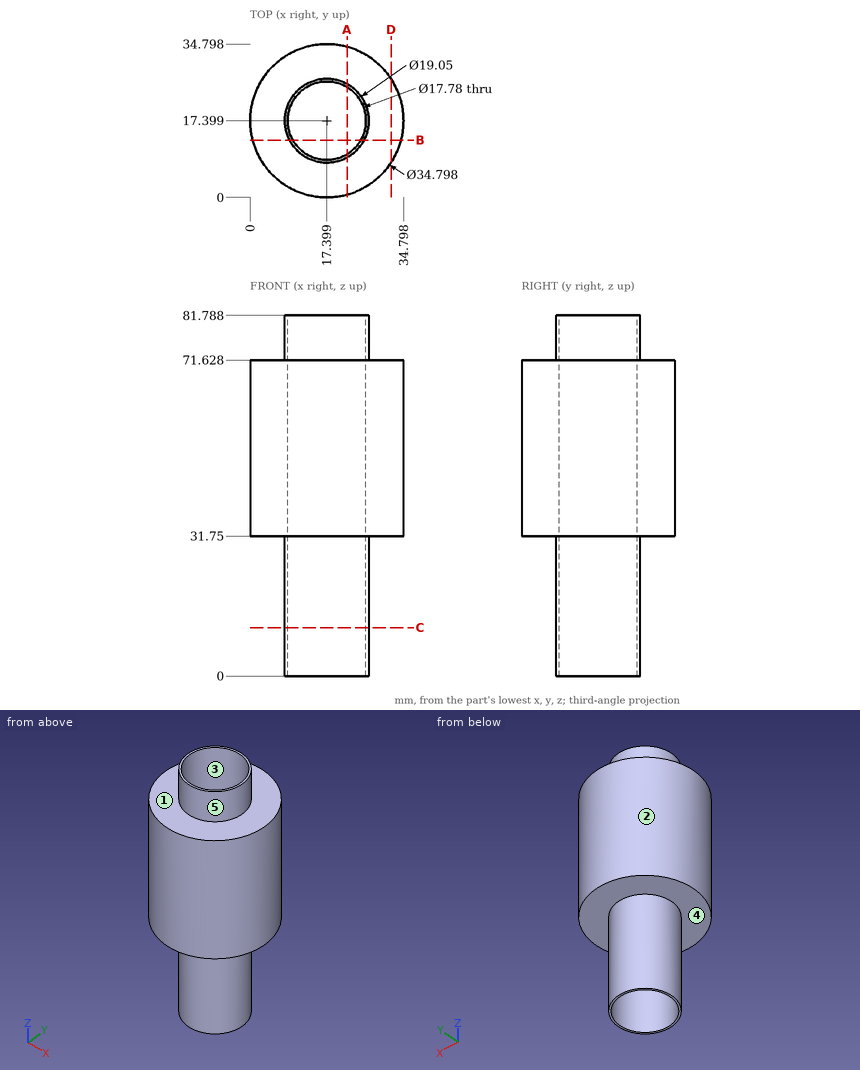
Design review of the part shown in the three views and the two pictorial views. Dimensions are in mm from the part's minimum x, y and z. A direction names the side the tool comes from. Coordinates: 2 decimals unless noted, no trailing zeros. Loops run counter-clockwise (first coordinate to the right, second up) from the corner with the lowest first, then second, coordinate; pieces in that order, holes last. Notation, with made-up numbers: M 39,50 L 49,50 A20 ccw 49,75 Z; hole C 64,-9 d11. An arc over 180 degrees is marked long. Put each result on its own line as item: value. Start each with the question number.
Q1. For the marked faces 4 and 5, list the 3-axis set-ups (+Z, -Z, +X, -X, +Y, -Y) from which the entire face can be reached by the end or side of a thin tool; tool diameter is ignored.
Q2. Add section A-A (x = 22). Write out the cut boundary in (y, z).
Q3. Add section D-D (x = 32). Write out the cut boundary in (y, z).
Q4. Add section C-C (z = 11). Write out the cut boundary in (x, y) (3 decimals).
Q5. Wall thickness on line 1 (Z direction, x = 22.5, y = 29.5); line 2 (Y direction, x = 12.5, z = 74); line 3 (Y direction, x = 23.5, z = 73): over which ranges is each line inside the solid? List them lowest first.
Q6. The part is to be moulded in two halves that separate along Y. For the marked faces 1, 2 and 3, say which applies: +Y half, -Y half, draft (parallel to the pull), parting line (faces both ways), or undercut.
Q7. Clearance check with flat-ended pins moving along their axes: pin 1 (10 mm diameter, centred on y = 25.5, z = 20.5, fed in from -X); pin 2 (2 mm diameter, centred on y = 4, z = 33.5, fed in from -X); pin 3 (16 mm diameter, centred on x = 17.399, y = 17.399, fed in from +Z); pin 4 (8 mm diameter, centred on x = 22, z = 15.5, fed in from -Y). State where each tip first meets the part, or that it passes through.
Q8. Add section B-B (y = 13). Write out the cut boundary in (x, z), and give its area (3 significant figures).
Answers:
1. face 4: -Z
1. face 5: +Z
2. outline: M 0.62,31.75 L 9.06,31.75 L 9.06,0 L 9.79,0 L 9.79,81.79 L 9.06,81.79 L 9.06,71.63 L 0.62,71.63 Z; M 25.01,0 L 25.74,0 L 25.74,31.75 L 34.18,31.75 L 34.18,71.63 L 25.74,71.63 L 25.74,81.79 L 25.01,81.79 Z
3. outline: M 7.94,31.75 L 26.86,31.75 L 26.86,71.63 L 7.94,71.63 Z
4. outline: C 17.399,17.399 d19.05; hole C 17.399,17.399 d17.78
5. line 1: z = 31.75 to 71.63
5. line 2: y = 9.23 to 9.98, 24.82 to 25.57
5. line 3: y = 10.08 to 10.93, 23.87 to 24.71
6. face 1: draft
6. face 2: parting line
6. face 3: undercut
7. pin 1: stops at x = 8.39
7. pin 2: stops at x = 5.19
7. pin 3: passes through
7. pin 4: stops at y = 7.89
8. outline: M 0.57,31.75 L 8.95,31.75 L 8.95,0 L 9.67,0 L 9.67,81.79 L 8.95,81.79 L 8.95,71.63 L 0.57,71.63 Z; M 25.12,0 L 25.85,0 L 25.85,31.75 L 34.23,31.75 L 34.23,71.63 L 25.85,71.63 L 25.85,81.79 L 25.12,81.79 Z
8. area: 787 mm^2
